The listing builds one solid part. Answer for the finished solid, in the listing's coordinates (mm). A direction names the side the tool comes from. Give positions to 0.01 mm unless a question says otherwise; leave off trailing zeros. Write each loop counter-clockwise with the first axis right and the second up, starting at its lowest first coordinate (ties: lowest second). Pieces come first, ordered by that corner, then holes. Notation, with made-up numbers: M 67,51.25 L 71,51.25 A24 ccw 71,71.25 Z; hole C 4,61 d2. An arc over 180 degrees is marked long. Return JSON: item names as keys, results as strings.
from build123d import *

# Parameters (mm, degrees)
SKETCH1_W           = 400
SKETCH1_H           = 420
BOSS_EXTRUDE1_DEPTH = 15
SKETCH2_R           = 25
CUT_EXTRUDE1_DEPTH  = 15
SKETCH3_W           = 50
SKETCH3_H           = 10
BOSS_EXTRUDE2_DEPTH = 230


with BuildPart() as part:
    # Sketch1 → Boss-Extrude1 (new body)
    with BuildSketch(Plane(origin=(0, 0, 0), x_dir=(1, 0, 0), z_dir=(0, 1, 0))):
        Rectangle(SKETCH1_W, SKETCH1_H)
    extrude(amount=BOSS_EXTRUDE1_DEPTH)

    # Sketch2 → Cut-Extrude1 (cut)
    with BuildSketch(Plane(origin=(0, 15, 0), x_dir=(1, 0, 0), z_dir=(0, 1, 0))):
        with Locations((-170, 180)):
            Circle(SKETCH2_R)
        with Locations((-170, -180)):
            Circle(SKETCH2_R)
        with Locations((170, -105)):
            Circle(SKETCH2_R)
        with Locations((170, 105)):
            Circle(SKETCH2_R)
    extrude(amount=-CUT_EXTRUDE1_DEPTH, mode=Mode.SUBTRACT)

    # Sketch3 → Boss-Extrude2 (add)
    with BuildSketch(Plane.XZ):
        with Locations((-95, 195)):
            Rectangle(SKETCH3_W, SKETCH3_H)
        with Locations((95, 195)):
            Rectangle(SKETCH3_W, SKETCH3_H)
        with Locations((-95, -195)):
            Rectangle(SKETCH3_W, SKETCH3_H)
        with Locations((95, -195)):
            Rectangle(SKETCH3_W, SKETCH3_H)
    extrude(amount=BOSS_EXTRUDE2_DEPTH)


solid = part.part
Item 1: A cutting plane is placed at A-A, the plane x = -170. Write down the section's boundary in (y, z), plus the area to 3 significant figures.
Geometry results:
{"outline": "M 0,-210 L 15,-210 L 15,-205 L 0,-205 Z; M 0,-155 L 15,-155 L 15,155 L 0,155 Z; M 0,205 L 15,205 L 15,210 L 0,210 Z", "area": "4,800 mm2"}
Item 2: Which of the six approach directions +Z, -Z, +X, -X, +Y, -Y give full straight-line access (tool end or side, diameter ignored) to faces 4 (the flat face through (120, -113, -195)), 5 (the flat face through (-95, -113, 190)), 6 (the flat face through (70, -113, 195))?
Geometry results:
{"face 4": "+Z, -Z, +X, -Y", "face 5": "+X, -X, -Y", "face 6": "+Z, -Z, -Y"}
Item 3: Given pin 1 Ø15 at (x, y) = (-96, -148.5) entering from -Z; pin 2 Ø5 at (y, z) = (-65, 192.5) entering from -X; pin 3 Ø25 at (x, y) = (91.5, -134) entering from +Z, each flat-ended and moving along its own axis, determine where each tip first touches the part or whether it passes through.
Geometry results:
{"pin 1": "stops at z = -200", "pin 2": "stops at x = -120", "pin 3": "stops at z = 200"}
Item 4: A cutting plane is placed at D-D, the plane x = -85.5. Write down the section's boundary in (y, z), plus the area to 3 significant figures.
Geometry results:
{"outline": "M -230,-200 L 0,-200 L 0,-210 L 15,-210 L 15,210 L 0,210 L 0,200 L -230,200 L -230,190 L 0,190 L 0,-190 L -230,-190 Z", "area": "10,900 mm2"}
Item 5: Determine the mould class of faces 1 (the flat face through (-200, 7, 3)), 2 (the flat face through (120, -113, 195)), 3 (the flat face through (-70, -113, -195)) for opening direction X: +X half, -X half, draft (parallel to the pull), parting line (faces both ways), or undercut.
Geometry results:
{"face 1": "-X half", "face 2": "+X half", "face 3": "undercut"}
Item 6: A cutting plane is placed at B-B, the plane y = -164.5. Write down the section's boundary in (x, z), plus the area to 3 significant figures.
Geometry results:
{"outline": "M -120,-200 L -70,-200 L -70,-190 L -120,-190 Z; M -120,190 L -70,190 L -70,200 L -120,200 Z; M 70,-200 L 120,-200 L 120,-190 L 70,-190 Z; M 70,190 L 120,190 L 120,200 L 70,200 Z", "area": "2,000 mm2"}
Item 7: Find the intervals of material crossed by line 1 (Z direction, x = 170, y = 4); line 2 (Z direction, x = -89.5, y = -12.5); line 3 (Y direction, x = -136, z = -155), in increasing order.
Geometry results:
{"line 1": "z = -210 to -130, -80 to 80, 130 to 210", "line 2": "z = -200 to -190, 190 to 200", "line 3": "y = 0 to 15"}
Item 8: A cutting plane is placed at C-C, the plane z = 105. Write down the section's boundary in (x, y), plus the area to 3 significant figures.
Geometry results:
{"outline": "M -200,0 L 145,0 L 145,15 L -200,15 Z; M 195,0 L 200,0 L 200,15 L 195,15 Z", "area": "5,250 mm2"}
